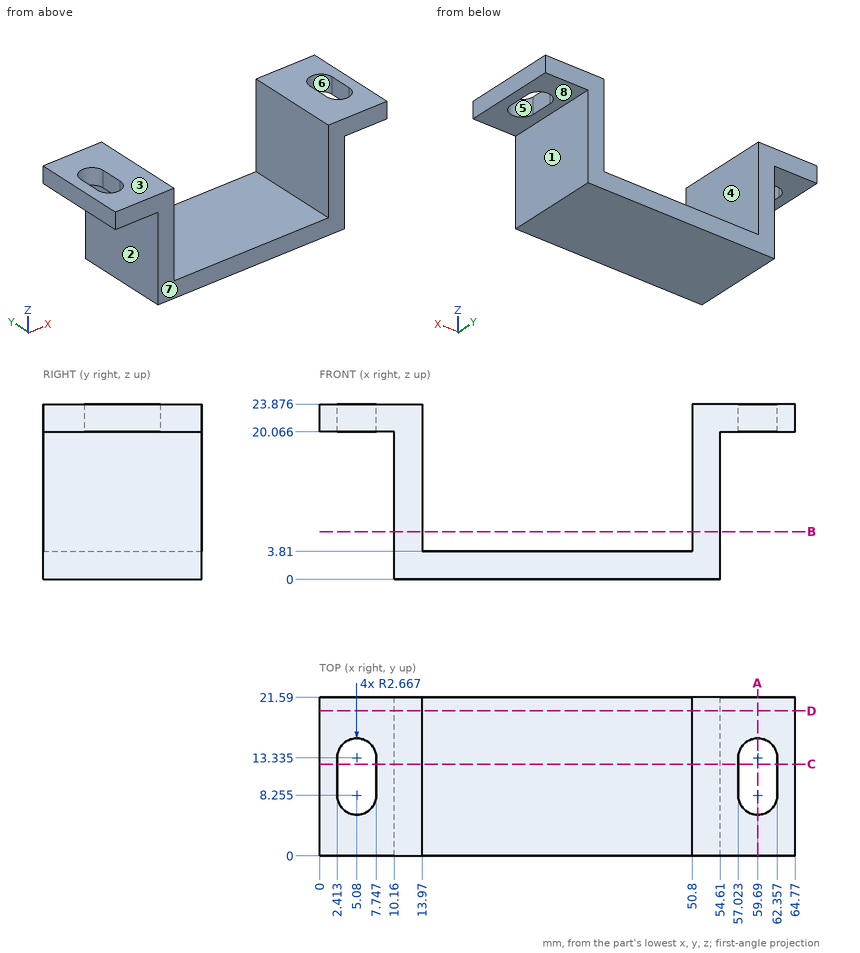
Job drawing, mm, ordinate dimensions from the low corner. One solid piece. A direction names the side the tool comes from. Give positions to 0.01 mm unless a question says otherwise; leave off trailing zeros. Loops run counter-clockwise (first coordinate to the right, second up) from the corner with the lowest first, then second, coordinate; pieces in that order, holes last. Notation, with made-up numbers: M 55.25,61.25 L 81.25,61.25 A28 ccw 81.25,89.25 Z; hole C -18,-38 d1. An arc over 180 degrees is marked long. Use one line per item in the form item = value.
Item 1: Two-plate mould, pull along Y, no slides. Class the marked faces 6, 7 and 8: released by +Y, released by -Y, zero draft, split by the parting line, or undercut.
Filled in:
face_6 = undercut
face_7 = released by -Y
face_8 = zero draft
Item 2: Slice it at B-B on z = 6.5. List the corners of the cut face in (x, y).
Filled in:
outline = M 10.16,0 L 13.97,0 L 13.97,21.59 L 10.16,21.59 Z; M 50.8,0 L 54.61,0 L 54.61,21.59 L 50.8,21.59 Z
Item 3: Slice it at C-C on y = 12.5. List the corners of the cut face in (x, z), and give its area (3 significant figures).
Filled in:
outline = M 0,20.07 L 2.41,20.07 L 2.41,23.88 L 0,23.88 Z; M 7.75,20.07 L 10.16,20.07 L 10.16,0 L 54.61,0 L 54.61,20.07 L 57.02,20.07 L 57.02,23.88 L 50.8,23.88 L 50.8,3.81 L 13.97,3.81 L 13.97,23.88 L 7.75,23.88 Z; M 62.36,20.07 L 64.77,20.07 L 64.77,23.88 L 62.36,23.88 Z
area = 359 mm^2
Item 4: Drill centre lines: L1, parallel to X at y = 5, z = 15.5; L2, parallel to X at y = 18.5, z = 22.75; L3, parallel to X at y = 7, z = 20.25. Where is each one in solid material? Low to high.
Filled in:
L1 = 10.16 to 13.97, 50.8 to 54.61
L2 = 0 to 13.97, 50.8 to 64.77
L3 = 0 to 2.73, 7.43 to 13.97, 50.8 to 57.34, 62.04 to 64.77
Item 5: Slice it at A-A on x = 59.69. List the corners of the cut face in (y, z), and give its area (3 significant figures).
Filled in:
outline = M 0,20.07 L 5.59,20.07 L 5.59,23.88 L 0,23.88 Z; M 16,20.07 L 21.59,20.07 L 21.59,23.88 L 16,23.88 Z
area = 42.6 mm^2
Item 6: Flat gauge pins, fed straight in: pin 1 Ø10 at (y, z) = (6.5, 10) entering from -X; pin 2 Ø6 at (y, z) = (4.5, 16.5) entering from +X; pin 3 Ø5 at (x, y) = (6.5, 7) entering from -Z. Where does each tip first touch, or does it go through?
Filled in:
pin_1 = 10.16
pin_2 = 54.61
pin_3 = 20.07
Item 7: Slice it at D-D on y = 19.75. List the corners of the cut face in (x, z), and give its area (3 significant figures).
Filled in:
outline = M 0,20.07 L 10.16,20.07 L 10.16,0 L 54.61,0 L 54.61,20.07 L 64.77,20.07 L 64.77,23.88 L 50.8,23.88 L 50.8,3.81 L 13.97,3.81 L 13.97,23.88 L 0,23.88 Z
area = 400 mm^2
Item 8: Which spindle directions (+Z, -Z, +X, -X, +Y, -Y) get a long thin tool onto all of the face, cutting with end or side? Do the marked faces 1, 2, 3, 4 and 5. Say none if no direction does.
Filled in:
face_1 = -Z, +X, +Y, -Y
face_2 = -Z, -X, +Y, -Y
face_3 = +Z, +X, -X, +Y, -Y
face_4 = +Z, +Y, -Y
face_5 = +Z, -Z
